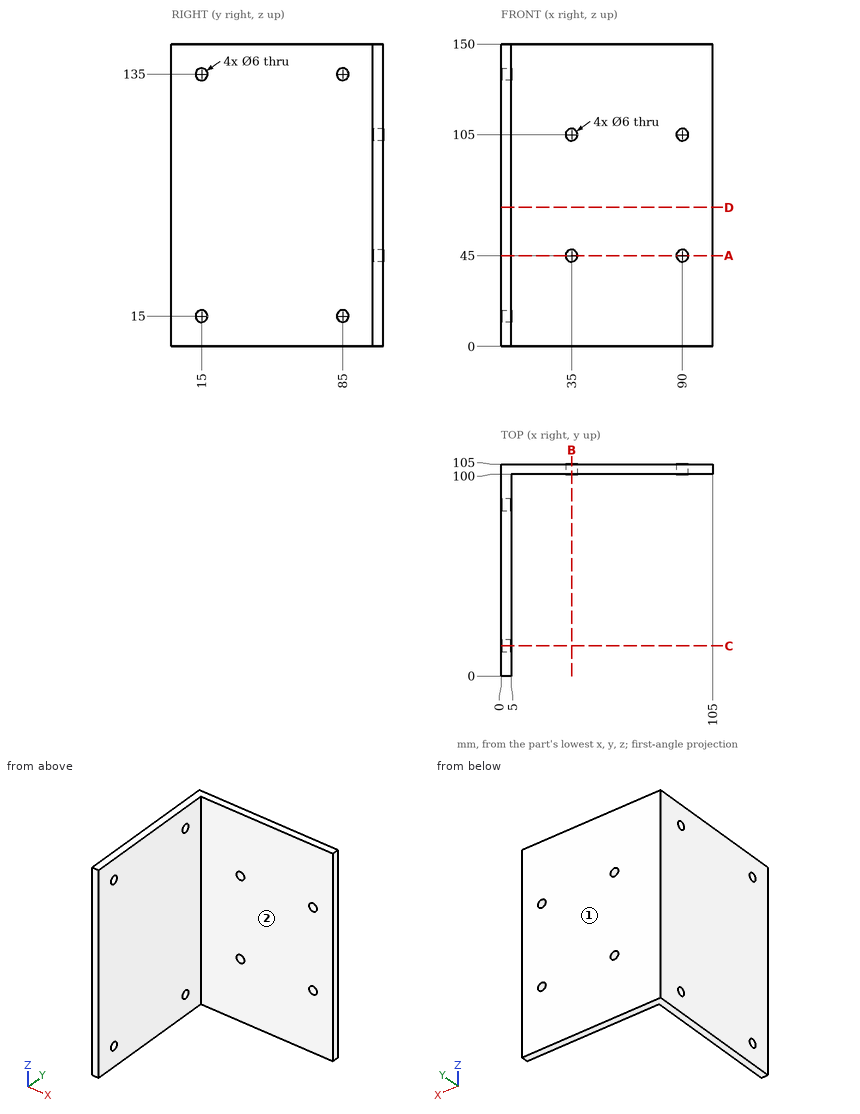
Can you work these out from the drawing? Everything is in mm from the part's minimum corner. A direction names the side the tool comes from. Round coordinates to 2 decimals unless told otherwise and drop trailing zeros. Order: outer loops, then holes, each group sorted by start corner. A loop starts at its lowest first (then second) coordinate and runs counter-clockwise, first axis right, second up. Notation, with made-up numbers: (-39.75, -39.75) - (1.25, -39.75) arc R22 ccw to (1.25, -21.75) - close; hole circle Ø8 at (22.25, -0.75). An arc over 180 degrees is marked (long way). Answer in a Markdown table with one row per item.
(1) Which directions (+Z, -Z, +X, -X, +Y, -Y) give clear straight access to the entire face, cutting with the end or side of a thin tool? Please do the marked faces 1 and 2.
From the geometry:
| item | result |
|---|---|
| face 1 | +Z, -Z, +X, -X, +Y |
| face 2 | +Z, -Z, +X, -Y |
(2) Suppose I cut it at A-A, the plane z = 45. Please give me the cut outline in (x, y).
From the geometry:
| item | result |
|---|---|
| outline | (0, 0) - (5, 0) - (5, 100) - (32, 100) - (32, 105) - (0, 105) - close; (38, 100) - (87, 100) - (87, 105) - (38, 105) - close; (93, 100) - (105, 100) - (105, 105) - (93, 105) - close |
(3) Suppose I cut it at B-B, the plane x = 35. Please give me the cut outline in (y, z).
From the geometry:
| item | result |
|---|---|
| outline | (100, 0) - (105, 0) - (105, 42) - (100, 42) - close; (100, 48) - (105, 48) - (105, 102) - (100, 102) - close; (100, 108) - (105, 108) - (105, 150) - (100, 150) - close |
(4) Please list where these lines run through material, in increasing order: L1, parallel to Z at x = 90, y = 102; L2, parallel to X at y = 66, z = 35.5; L3, parallel to Y at x = 83.5, z = 126.5. Write a range as from..to.
From the geometry:
| item | result |
|---|---|
| L1 | z = 0..42, 48..102, 108..150 |
| L2 | x = 0..5 |
| L3 | y = 100..105 |
(5) For P1, Ø12, axis at y = 85.5, z = 26.5, coming from the +X side; P2, Ø7, axis at x = 35, z = 105, coming from the -Y side, each with a flat end and sliding along its axis, tell me the tip position at first contact or that it passes through.
From the geometry:
| item | result |
|---|---|
| P1 | stops at x = 5 |
| P2 | stops at y = 100 |
(6) Suppose I cut it at D-D, the plane z = 69. Please give me the cut outline in (x, y).
From the geometry:
| item | result |
|---|---|
| outline | (0, 0) - (5, 0) - (5, 100) - (105, 100) - (105, 105) - (0, 105) - close |
(7) Suppose I cut it at C-C, the plane y = 15. Please give me the cut outline in (x, z), plus the area to 3 significant figures.
From the geometry:
| item | result |
|---|---|
| outline | (0, 0) - (5, 0) - (5, 12) - (0, 12) - close; (0, 18) - (5, 18) - (5, 132) - (0, 132) - close; (0, 138) - (5, 138) - (5, 150) - (0, 150) - close |
| area | 690 mm2 |
